Work out the finished part from the listing and answer in its coordinate system (mm). A direction names the side the tool comes from. Coordinates: 2 decimals unless noted, no trailing zeros. Order: outer loops, then holes, each group sorted by start corner. A loop starts at its lowest first (then second) coordinate and runs counter-clockwise, first axis right, second up. Notation, with made-up numbers: M -30,-22 L 11,-22 A30 cw 11,10 Z; hole C -3,77.25 d3. An arc over 180 degrees is marked long. Answer in a Markdown table with one row per item. Add a question column.
Item 1: Which of the six approach directions +Z, -Z, +X, -X, +Y, -Y give full straight-line access (tool end or side, diameter ignored) to faces 5 (the face through (7.5, 1, 0)), 6 (the face through (7, 10.5, 0)), 7 (the face through (7.885, 5.325, 0.013)), 8 (the face through (6.418, 9.526, 0.013)), 9 (the face through (4.05, 2.27, 0.01))?
Item 2: The part is cut by section B-B (z = 0.75). Write down the section's boundary in (x, y), then the cut area to 3 significant figures.
Item 3: The part is cut by section C-C (y = 6.5). Write down the section's boundary in (x, z).
Item 4: The mould has two halves that part along Y. Classify faces 1 (the face through (6, 6, 0)), 2 (the face through (3, 1, 0)), 3 (the face through (5, 0, 0)), 4 (the face through (7, 4, 0.9)): released by +Y, released by -Y, zero draft, split by the parting line, or undercut.
Item 5: The part is cut by section A-A (x = 7.25). Write down the section's boundary in (y, z), then the cut area to 3 significant figures.
Item 6: Consider line 1 (X direction, y = 6.5, z = -0.1); line 2 (Y direction, x = 6.75, z = -0.25); line 3 (X direction, y = 4.75, z = -0.1). Determine where each line is inside the solid, lowest interval first. Write a range as from..to.
Item 7: The part is cut by section D-D (x = 2.5). Write down the section's boundary in (y, z), then the cut area to 3 significant figures.
from build123d import *

# Parameters (mm, degrees)
F1_DEPTH = 0.9
F2_R     = 8
F2_R_2   = 7.5
F3_DEPTH = 2


with BuildPart() as f1:
    # F0 (on Top) → F1 (new body, symmetric)
    with BuildSketch(Plane.XY):
        with BuildLine():
            Line((2, 0), (7.5, 0))
            Line((7.5, 0), (7.5, 2))
            Line((7.5, 2), (6.480741, 2))
            ThreePointArc((6.480741, 2), (6.113547, 2.241354), (6.189471, 2.674157))
            ThreePointArc((6.189471, 2.674157), (7.901282, 5.366353), (8.5, 8.5))
            Line((8.5, 8.5), (6.5, 8.5))
            ThreePointArc((6.5, 8.5), (5.897033, 5.765955), (4.2, 3.539153))
            Line((4.2, 3.539153), (4.2, 3.028427))
            ThreePointArc((4.2, 3.028427), (4.047759, 2.26306), (3.614214, 1.614214))
            Line((3.614214, 1.614214), (2, 0))
        make_face()
        with BuildLine():
            Line((6.5, 8.5), (8.5, 8.5))
            ThreePointArc((8.5, 8.5), (8.440128, 9.507094), (8.261356, 10.5))
            Line((8.261356, 10.5), (6.184658, 10.5))
            ThreePointArc((6.184658, 10.5), (6.420681, 9.512354), (6.5, 8.5))
        make_face()
    extrude(amount=F1_DEPTH, both=True)

    # F2 (on face) → F3 (cut, through all)
    with BuildSketch(Plane.XZ):
        Circle(F2_R)
        Circle(F2_R_2, mode=Mode.SUBTRACT)
    extrude(amount=-F3_DEPTH, mode=Mode.SUBTRACT)


solid = f1.part
Reply:
| question | item | result |
|---|---|---|
| 1 | face 5 | +X, -Y |
| 1 | face 6 | +Z, -Z, +X, -X, +Y |
| 1 | face 7 | +Z, -Z, +X |
| 1 | face 8 | +Z, -Z, -X |
| 1 | face 9 | +Z, -Z, -X, +Y |
| 2 | outline | M 2,0 L 7.46,0 L 7.46,2 L 6.48,2 A0.4 cw 6.19,2.67 A8.5 ccw 8.5,8.5 A8.5 ccw 8.26,10.5 L 6.18,10.5 A6.5 cw 6.5,8.5 A6.5 cw 4.2,3.54 L 4.2,3.03 A2 cw 3.61,1.61 Z |
| 2 | area | 27.3 mm2 |
| 3 | outline | M 6.18,-0.9 L 8.26,-0.9 L 8.26,0.9 L 6.18,0.9 Z |
| 4 | face 1 | undercut |
| 4 | face 2 | released by +Y |
| 4 | face 3 | released by -Y |
| 4 | face 4 | zero draft |
| 5 | outline | M 0,-0.9 L 2,-0.9 L 2,0.9 L 0,0.9 Z; M 4.06,-0.9 L 10.5,-0.9 L 10.5,0.9 L 4.06,0.9 Z |
| 5 | area | 15.2 mm2 |
| 6 | line 1 | x = 6.18..8.26 |
| 6 | line 2 | y = 0..2, 3.33..10.5 |
| 6 | line 3 | x = 5.31..7.63 |
| 7 | outline | M 0,-0.9 L 0.5,-0.9 L 0.5,0.9 L 0,0.9 Z |
| 7 | area | 0.900 mm2 |
